Design review of the part built by this model. Coordinates are the model's own, in mm. A direction names the side the tool comes from. Coordinates: 2 decimals unless noted, no trailing zeros. Write each loop counter-clockwise with the first axis right and the second up, starting at its lowest first coordinate (ties: lowest second). Pieces come first, ordered by that corner, then holes.
Q1. For probe 1 along Z at (x, y) = (0, 6.75); probe 2 along X at (y, z) = (5, 1.5) (3 decimals); probe 3 along Z at (x, y) = (0.5, -5), list the stretches that pass through material, from the lowest coordinate up.
Q2. Take a section at B-B (y = -4.25). Give the boundary of the cut face in (x, z), and give its area (3 significant figures).
Q3. Insertion check: pin 1 (3.5 mm diameter, centred on y = 0.5, z = 14, fed in from +X); pin 2 (3 mm diameter, centred on x = -3, z = 6, fed in from +Y); pin 3 (4.5 mm diameter, centred on x = 3.5, z = 4.5, fed in from -Y); pin 4 (6.5 mm diameter, centred on x = 0, y = 3, fed in from +Z). Each pin has a flat end and moves straight along its axis. Give the tip position at first contact, or say it passes through.
Q4. Take a section at A-A (z = 3). Give the boundary of the cut face in (x, y), and give its area (3 significant figures).
Q5. Machinability: for faces 1 (the flat face through (0, 0, 10)), 2 (the cylindrical face through (0.11, -2.57, 0.6)), 3 (the flat face through (0, 6, 0)), which of the approach directions +Z, -Z, +X, -X, +Y, -Y give a long, thin tool a straight path to every point of the face, cutting with its end or side? Answer none if there is none.
Q6. Mouldability with a two-part tool opening along Y and no side actions: class faces 4 (the cylindrical face through (7.39, -3.06, 7.48)), 5 (the cylindrical face through (-4.4, -0.1, 10.57)), 6 (the cylindrical face through (-6, 0, 15)), 7 (the flat face through (-0.1, -2, 4.4)) as pulls with the +Y half, pulls with the -Y half, needs draft (parallel to the pull), parting line crosses it, or undercut.
Q7. Take a section at D-D (z = 13.5). Give the boundary of the cut face in (x, y) (3 decimals), and give its area (3 significant figures).
```python
from build123d import *

# Parameters (mm, degrees)
F0_R         = 8
F1_DEPTH     = 20
F3_DEPTH     = 10
F5_DEPTH     = 8
F7_D         = 2
F7_DEPTH     = 3.001
F9_D         = 2
F10_T1_DEPTH = 37.4894960018
F12_D        = 2
F12_DEPTH    = 6.0010001
F14_D        = 2
F15_R        = 2
F16_R        = 1.9999


# Not quite as in the source:
# - a fillet or chamfer that OpenCascade refuses, or shapes differently, is made with other operations: its cross-section is extruded or revolved along the edge and cut away or added
# - a fillet or chamfer is up to 0.001 mm smaller than in the source, because OpenCascade refuses the exact size


with BuildPart() as f1:
    # F0 (on Top) → F1 (new body)
    with BuildSketch(Plane.XY):
        Circle(F0_R)
    extrude(amount=F1_DEPTH)

    # F2 (on face) → F3 (cut)
    with BuildSketch(Plane.XY.offset(20)):
        with BuildLine():
            ThreePointArc((5, 6.2449979984), (0, 8), (-5, 6.2449979984))
            Line((-5, 6.2449979984), (-5, -6.2449979984))
            ThreePointArc((-5, -6.2449979984), (0, -8), (5, -6.2449979984))
            Line((5, -6.2449979984), (5, 6.2449979984))
        make_face()
    extrude(amount=-F3_DEPTH, mode=Mode.SUBTRACT)

    # F4 (on face) → F5 (cut)
    with BuildSketch(Plane.XY):
        with BuildLine():
            ThreePointArc((8, 0), (7.9362375701, 1.0080343399), (7.7459666924, 2))
            Line((7.7459666924, 2), (-7.7459666924, 2))
            ThreePointArc((-7.7459666924, 2), (-7.9362375701, 1.0080343399), (-8, 0))
            ThreePointArc((-8, 0), (-7.9362375701, -1.0080343399), (-7.7459666924, -2))
            Line((-7.7459666924, -2), (7.7459666924, -2))
            ThreePointArc((7.7459666924, -2), (7.9362375701, -1.0080343399), (8, 0))
        make_face()
    extrude(amount=F5_DEPTH, mode=Mode.SUBTRACT)

    # F7 (through all, one way)
    with BuildSketch(Plane.YZ.offset(-5)):
        with Locations((0, 16)):
            Circle(F7_D / 2)
    extrude(amount=-F7_DEPTH, mode=Mode.SUBTRACT)

    # F9 (through all)
    with Locations(Plane(origin=(5, 0, 0), x_dir=(0, -1, 0), z_dir=(-1, 0, 0))):
        with Locations((0, 16)):
            Hole(F9_D / 2)

    # F10: fillet of radius 5 on 2 edges, made by hand

    # F10_s2 → F10_t1 (cut)
    with BuildSketch(Plane.XZ.offset(-18.7447480009)):
        with BuildLine():
            ThreePointArc((9.9999, 20.0001), (6.4643660941, 18.5356339059), (4.9999, 15.0001))
            Line((4.9999, 15.0001), (4.8999, 15.0001))
            ThreePointArc((4.8999, 15.0001), (4.9, 17.50005), (4.9, 20))
            Line((4.9, 20), (5, 20.1))
            ThreePointArc((5, 20.1), (7.49995, 20.1), (9.9999, 20.1001))
            Line((9.9999, 20.1001), (9.9999, 20.0001))
        make_face()
        with BuildLine():
            ThreePointArc((-4.9999, 15.0001), (-6.4643660941, 18.5356339059), (-9.9999, 20.0001))
            Line((-9.9999, 20.0001), (-9.9999, 20.1001))
            ThreePointArc((-9.9999, 20.1001), (-7.49995, 20.1), (-5, 20.1))
            Line((-5, 20.1), (-4.9, 20))
            ThreePointArc((-4.9, 20), (-4.9, 17.50005), (-4.8999, 15.0001))
            Line((-4.8999, 15.0001), (-4.9999, 15.0001))
        make_face()
    extrude(amount=F10_T1_DEPTH, mode=Mode.SUBTRACT)

    # F12 (through all, one way)
    with BuildSketch(Plane(origin=(0, -2, 0), x_dir=(-1, 0, 0), z_dir=(0, 1, 0))):
        with Locations((0, 3)):
            Circle(F12_D / 2)
    extrude(amount=-F12_DEPTH, mode=Mode.SUBTRACT)

    # F14 (through all)
    with Locations(Plane.XZ.offset(-2)):
        with Locations((0, 3)):
            Hole(F14_D / 2)

    # F15
    f15_edges = [f1.edges().sort_by_distance(p)[0] for p in [
        (0, 2, 0),
        (0, -2, 0),
    ]]
    fillet(f15_edges, radius=F15_R)

    # F16 (radius 2 in the source; OpenCascade refuses exactly that, so slightly less here)
    f16_edges = [f1.edges().sort_by_distance(p)[0] for p in [
        (-5, 0, 10),
        (5, 0, 10),
        (0, 2, 8),
        (0, -2, 8),
    ]]
    fillet(f16_edges, radius=F16_R)


solid = f1.part
```
Response:
1. probe 1: z = 0 to 2, 4 to 10
1. probe 2: x = -6.245 to 6.245
1. probe 3: z = 0 to 2.13, 3.87 to 10
2. outline: (-6.78, 0) - (6.78, 0) - (6.78, 18.82) arc R5 ccw to (5, 15.03) - (5, 12) arc R2 cw to (3, 10) - (-3, 10) arc R2 cw to (-5, 12) - (-5, 15.03) arc R5 ccw to (-6.78, 18.82) - close; hole circle Ø2 at (0, 3)
2. area: 161 mm2
3. pin 1: stops at x = 8
3. pin 2: stops at y = 7.86
3. pin 3: stops at y = -7.9
3. pin 4: stops at z = 10.02
4. outline: (-7.75, -2) arc R8 ccw to (-1, -7.94) - (-1, -2) - close; (-7.75, 2) - (-1, 2) - (-1, 7.94) arc R8 ccw to start; (1, -7.94) arc R8 ccw to (7.75, -2) - (1, -2) - close; (1, 2) - (7.75, 2) arc R8 ccw to (1, 7.94) - close
4. area: 114 mm2
5. face 1: +Z, +Y, -Y
5. face 2: -Z, +X, -X
5. face 3: -Z, +X, -X, +Y, -Y
6. face 4: parting line crosses it
6. face 5: needs draft
6. face 6: undercut
6. face 7: undercut
7. outline: (-5, -6.245) - (-5, 6.245) arc R8 ccw to start; (5, -6.245) arc R8 ccw to (5, 6.245) - close
7. area: 52.2 mm2
